```python
from build123d import *

# Parameters (mm, degrees)
SKETCH_2_R          = 30
EXTRUDE_1_DEPTH     = 70
SKETCH_3_R          = 20
CUT_EXTRUDE_2_DEPTH = 15
CUT_EXTRUDE_3_DEPTH = 55
EXTRUDE_START       = 43
EXTRUDE_2_DEPTH     = 15
SKETCH_7_R          = 7.5
CUT_EXTRUDE_4_DEPTH = 15


with BuildPart() as part:
    # 草图2 → 凸台-拉伸1 (new body)
    with BuildSketch(Plane(origin=(0, 0, 0), x_dir=(1, 0, 0), z_dir=(0, 1, 0))):
        with Locations(Location((0, -1.173457716, 0), (0, 0, 270))):
            Circle(SKETCH_2_R)
    extrude(amount=EXTRUDE_1_DEPTH)

    # 草图3 → 切除-拉伸2 (cut)
    with BuildSketch(Plane(origin=(0, 70, 0), x_dir=(1, 0, 0), z_dir=(0, 1, 0))):
        with Locations(Location((0, 0, 0), (0, 0, 270))):
            Circle(SKETCH_3_R)
    extrude(amount=-CUT_EXTRUDE_2_DEPTH, mode=Mode.SUBTRACT)

    # 草图5 → 切除-拉伸3 (cut)
    with BuildSketch(Plane.XZ):
        Polygon((0, 12.727922061), (12.727922061, 0), (0, -12.727922061), (-12.727922061, 0), align=None)
    extrude(amount=-CUT_EXTRUDE_3_DEPTH, mode=Mode.SUBTRACT)

    # 草图6 → 凸台-拉伸2 (add)
    with BuildSketch(Plane(origin=(0, 0, 0), x_dir=(1, 0, 0), z_dir=(0, 1, 0)).offset(EXTRUDE_START)):
        with BuildLine():
            Line((-15, 50), (-15, 24.807304398))
            ThreePointArc((-15, 24.807304398), (0, 28.826542284), (15, 24.807304398))
            Line((15, 24.807304398), (15, 50))
            ThreePointArc((15, 50), (0, 65), (-15, 50))
        make_face()
    extrude(amount=EXTRUDE_2_DEPTH)

    # 草图7 → 切除-拉伸4 (cut)
    with BuildSketch(Plane(origin=(0, 58, 0), x_dir=(1, 0, 0), z_dir=(0, 1, 0))):
        with Locations(Location((0, 50, 0), (0, 0, 270))):
            Circle(SKETCH_7_R)
    extrude(amount=-CUT_EXTRUDE_4_DEPTH, mode=Mode.SUBTRACT)


solid = part.part
```
Can you work these out from the model? Positions are in its coordinate system, mm. A direction names the side the tool comes from. Give positions to 0.01 mm unless a question says otherwise; leave off trailing zeros. Write each loop counter-clockwise with the first axis right and the second up, starting at its lowest first coordinate (ties: lowest second). Pieces come first, ordered by that corner, then holes. Notation, with made-up numbers: (2.25, 80.25) -> (56.25, 80.25) arc R22 ccw to (56.25, 118.25) -> close; hole circle Ø10 at (52, -18). An arc over 180 degrees is marked (long way). Write item = value, one per line.
(1) Suppose I cut it at A-A on y = 45. Write out the boundary of the cut face in (x, z).
Worked out:
outline = (-15, -50) arc R15 ccw to (15, -50) -> (15, -24.81) arc R30 ccw (long way) to (-15, -24.81) -> close; hole (-12.73, 0) -> (0, -12.73) -> (12.73, 0) -> (0, 12.73) -> close; hole circle Ø15 at (0, -50)
(2) Thinking about a two-plate mould opening in X: for faces 5 (the face through (-11.49, 34.51, 28.886)), 6 (the face through (6.275, 27.115, 6.453)), 7 (the face through (0, 43, -41)), which applies, released by +X, released by -X, zero draft, split by the parting line, or undercut?
Worked out:
face_5 = split by the parting line
face_6 = undercut
face_7 = zero draft
(3) I need wall thicknesses on probe 1 along X at (y, z) = (66, 0); probe 2 along Z at (x, y) = (-2.5, 56.5); probe 3 along Y at (x, z) = (9, -33). Which ranges of each line are inside material? Lowest first, please. Write a range as from..to.
Worked out:
probe_1 = -29.98..-20, 20..29.98
probe_2 = -64.79..-57.07, -42.93..-19.84, 19.84..31.07
probe_3 = 43..58
(4) Suppose I cut it at D-D on x = 4.5. Write out the boundary of the cut face in (y, z).
Worked out:
outline = (0, -28.49) -> (43, -28.49) -> (43, -44) -> (58, -44) -> (58, -28.49) -> (70, -28.49) -> (70, -19.49) -> (55, -19.49) -> (55, -8.23) -> (0, -8.23) -> close; (0, 8.23) -> (55, 8.23) -> (55, 19.49) -> (70, 19.49) -> (70, 30.83) -> (0, 30.83) -> close; (43, -64.31) -> (58, -64.31) -> (58, -56) -> (43, -56) -> close
(5) I'm going to push flat-ended pins straight in: P1, Ø9, axis at x = -6.5, z = -40.5, coming from the -Y side; P2, Ø2, axis at y = 34, z = 12.5, coming from the -X side; P3, Ø12, axis at x = -23, z = 21, coming from the -Y side; P4, Ø1.5, axis at x = -21.5, y = 8, coming from the +Z side. Where does each tip first touch, or does it pass through?
Worked out:
P1 = 43
P2 = -28.17
P3 = 0
P4 = 22.84
(6) Suppose I cut it at B-B on z = -45. Write out the boundary of the cut face in (x, y).
Worked out:
outline = (-15, 43) -> (-5.59, 43) -> (-5.59, 58) -> (-15, 58) -> close; (5.59, 43) -> (15, 43) -> (15, 58) -> (5.59, 58) -> close
(7) Suppose I cut it at C-C on y = 35. Write out the boundary of the cut face in (x, z), then the cut area to 3 significant figures.
Worked out:
outline = circle Ø60 at (0, 1.17); hole (-12.73, 0) -> (0, -12.73) -> (12.73, 0) -> (0, 12.73) -> close
area = 2,500 mm^2
(8) For faces 1 (the face through (-6.453, 27.115, 6.275)), 2 (the face through (-19.524, 62.605, -4.336)), 3 (the face through (-15, 50, -38)), 4 (the face through (15, 50, -37)), which set-ups out of +Z, -Z, +X, -X, +Y, -Y let a thin tool reach every point of the face, with its end or its side?
Worked out:
face_1 = +Y, -Y
face_2 = +Y
face_3 = -Z, -X, +Y, -Y
face_4 = -Z, +X, +Y, -Y
